Job drawing, mm, ordinate dimensions from the low corner. One solid piece. Give positions to 0.01 mm unless a question says otherwise; leave off trailing zeros. Write each loop counter-clockwise with the first axis right and the second up, starting at its lowest first coordinate (ties: lowest second). Pieces come first, ordered by that corner, then holes. Notation, with made-up numbers: M 18,30.25 L 62,30.25 A20 ccw 62,56.25 Z; hole C 2,46 d4. An arc over 180 degrees is marked long. Use a Markdown table: item, result.
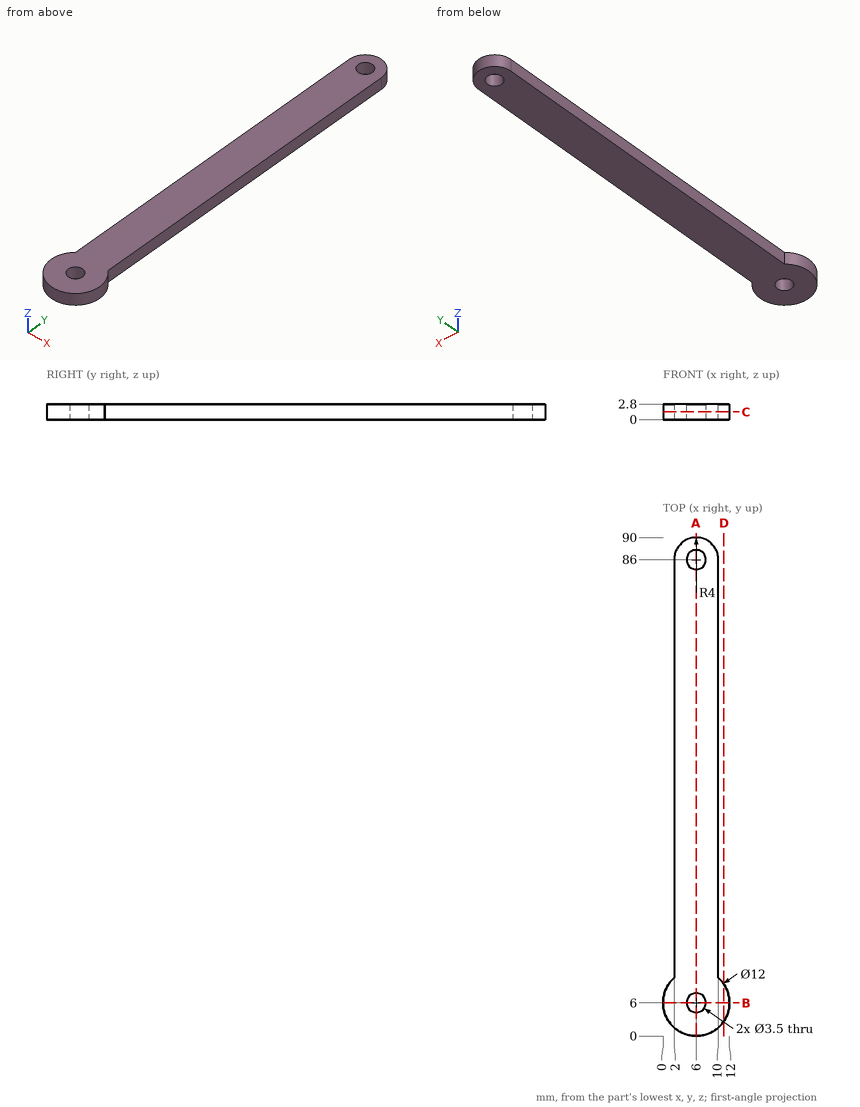
1. Cut at B-B, the plane y = 6. Give the cut face in (x, z).
Findings below:
| item | result |
|---|---|
| outline | M 0,0 L 4.25,0 L 4.25,2.8 L 0,2.8 Z; M 7.75,0 L 12,0 L 12,2.8 L 7.75,2.8 Z |
2. Cut at A-A, the plane x = 6. Give the cut face in (y, z), then the cut area to 3 significant figures.
Findings below:
| item | result |
|---|---|
| outline | M 0,0 L 4.25,0 L 4.25,2.8 L 0,2.8 Z; M 7.75,0 L 84.25,0 L 84.25,2.8 L 7.75,2.8 Z; M 87.75,0 L 90,0 L 90,2.8 L 87.75,2.8 Z |
| area | 232 mm2 |
3. Cut at D-D, the plane x = 11. Give the cut face in (y, z).
Findings below:
| item | result |
|---|---|
| outline | M 2.68,0 L 9.32,0 L 9.32,2.8 L 2.68,2.8 Z |
4. Drop flat-ended pins along their axis: P1, Ø1.5, axis at y = 56, z = 0.5, coming from the +X side; P2, Ø1.5, axis at y = 77, z = 0.5, coming from the -X side. Give the stop position or say it passes through.
Findings below:
| item | result |
|---|---|
| P1 | x = 10 |
| P2 | x = 2 |
5. Cut at C-C, the plane z = 1.4. Give the cut face in (x, y), then the cut area to 3 significant figures.
Findings below:
| item | result |
|---|---|
| outline | M 2,10.47 A6 ccw long 10,10.47 L 10,86 A4 ccw 2,86 Z; hole C 6,6 d3.5; hole C 6,86 d3.5 |
| area | 715 mm2 |
6. Drill centre lines: L1, parallel to Y at x = 6, z = 1.25; L2, parallel to X at y = 86, z = 1.5; L3, parallel to Y at x = 4.5, z = 2.2. Where is each one in solid material? Low to high.
Findings below:
| item | result |
|---|---|
| L1 | 0 to 4.25, 7.75 to 84.25, 87.75 to 90 |
| L2 | 2 to 4.25, 7.75 to 10 |
| L3 | 0.19 to 5.1, 6.9 to 85.1, 86.9 to 89.71 |
